```python
from build123d import *

# Parameters (mm, degrees)
F1_DEPTH = 2.54


with BuildPart() as f1:
    # F0 (on Front) → F1 (new body)
    with BuildSketch(Plane.XZ):
        with BuildLine():
            ThreePointArc((7.738306, -7.057663), (9.765713, -3.784552), (10.473394, 0))
            ThreePointArc((10.473394, 0), (9.627005, 4.124653), (7.224635, 7.582653))
            ThreePointArc((7.224635, 7.582653), (0, 10.473394), (-7.224635, 7.582653))
            ThreePointArc((-7.224635, 7.582653), (-10.466954, 0.367244), (-7.738306, -7.057663))
            ThreePointArc((-7.738306, -7.057663), (0, -10.473394), (7.738306, -7.057663))
        make_face()
        with BuildLine():
            Line((-2.152094, -7.214504), (0, -2.595979))
            Line((0, -2.595979), (2.144959, -7.214504))
            ThreePointArc((2.144959, -7.214504), (-0.003567, -7.636494), (-2.152094, -7.214504))
        make_face(mode=Mode.SUBTRACT)
        with BuildLine():
            ThreePointArc((-3.384339, -6.653862), (-6.683961, -3.233143), (-7.223777, 1.488871))
            Line((-7.223777, 1.488871), (-3.384339, -6.653862))
        make_face(mode=Mode.SUBTRACT)
        with BuildLine():
            Line((3.492318, -6.653862), (7.286586, 1.488871))
            ThreePointArc((7.286586, 1.488871), (6.822869, -3.250425), (3.492318, -6.653862))
        make_face(mode=Mode.SUBTRACT)
        with BuildLine():
            ThreePointArc((-5.957007, 4.418221), (-5.252536, 5.505791), (-4.134786, 6.161323))
            Line((-4.134786, 6.161323), (-1.229617, 0))
            Line((-1.229617, 0), (1.402125, 0))
            Line((1.402125, 0), (4.273116, 6.161323))
            ThreePointArc((4.273116, 6.161323), (5.263901, 5.39392), (6.050396, 4.418221))
            Line((6.050396, 4.418221), (2.601226, -2.98391))
            Line((2.601226, -2.98391), (1.402125, -0.328891))
            Line((1.402125, -0.328891), (-1.229617, -0.328891))
            Line((-1.229617, -0.328891), (-2.466776, -2.98391))
            Line((-2.466776, -2.98391), (-5.957007, 4.418221))
        make_face(mode=Mode.SUBTRACT)
        with BuildLine():
            Line((0, 2.846012), (-1.913186, 7.11832))
            ThreePointArc((-1.913186, 7.11832), (0.103343, 7.357841), (2.119873, 7.11832))
            Line((2.119873, 7.11832), (0, 2.846012))
        make_face(mode=Mode.SUBTRACT)
        with BuildLine():
            ThreePointArc((7.224635, 7.582653), (9.627005, 4.124653), (10.473394, 0))
            ThreePointArc((10.473394, 0), (9.765713, -3.784552), (7.738306, -7.057663))
            Line((7.738306, -7.057663), (17.044773, -4.823679))
            Line((17.044773, -4.823679), (17.261992, -4.200394))
            Line((17.261992, -4.200394), (21.515753, 8.005273))
            Line((21.515753, 8.005273), (9.83273, 7.65978))
            Line((9.83273, 7.65978), (7.224635, 7.582653))
        make_face()
        with BuildLine():
            ThreePointArc((-7.738306, -7.057663), (-10.466954, 0.367244), (-7.224635, 7.582653))
            Line((-7.224635, 7.582653), (-9.815511, 7.65978))
            Line((-9.815511, 7.65978), (-21.421401, 8.005273))
            Line((-21.421401, 8.005273), (-17.155705, -4.200394))
            Line((-17.155705, -4.200394), (-16.937877, -4.823679))
            Line((-16.937877, -4.823679), (-7.738306, -7.057663))
        make_face()
        Polygon((-14.769453, 2.473412), (-14.185613, 4.333009), (-13.477944, 2.473412), (-11.474869, 2.473412), (-13.129719, 1.022873), (-12.338734, -1.062449), (-14.252342, 0.338954), (-15.897308, -1.062449), (-15.132699, 1.022873), (-16.792862, 2.473412), align=None, mode=Mode.SUBTRACT)
        Polygon((11.004867, 10.780503), (9.83273, 7.65978), (21.515753, 8.005273), (17.261992, -4.200394), (44.487608, 2.368847), (50.83166, 10.780503), align=None)
        Polygon((-21.421401, 8.005273), (-9.815511, 7.65978), (-11.012142, 10.780503), (-50.76834, 10.780503), (-44.232576, 2.368847), (-17.155705, -4.200394), align=None)
    extrude(amount=F1_DEPTH)


solid = f1.part
```
The listing builds one solid part. Answer for the finished solid, in the listing's coordinates (mm). A direction names the side the tool comes from. Give positions to 0.01 mm unless a question says otherwise; leave off trailing zeros. Order: outer loops, then holes, each group sorted by start corner. A loop starts at its lowest first (then second) coordinate and runs counter-clockwise, first axis right, second up.
Item 1: Find the intervals of material crossed by probe 1 along X at (y, z) = (-1, 5.75); probe 2 along Z at (x, y) = (6, -0.6); probe 3 along Z at (x, y) = (1.5, -0.6), in increasing order.
From the geometry:
probe 1: x = -46.86 to -4.96, -3.94 to -1.3, 1.44 to 4.08, 4.86 to 47.04
probe 2: z = -8.58 to -4.6, -1.27 to 4.31, 4.5 to 8.58
probe 3: z = -10.37 to -7.43, -5.83 to -0.55, 0.21 to 5.87, 7.24 to 10.37
Item 2: The part is cut by section C-C, the plane x = 29.5. Give the vertices of the cut face in (y, z), and give its area (3 significant figures).
From the geometry:
outline: (-2.54, -1.25) - (0, -1.25) - (0, 10.78) - (-2.54, 10.78) - close
area: 30.6 mm2
Item 3: Given pin 1 Ø10 at (x, z) = (-5.5, -5) entering from +Y; pin 2 Ø0.6 at (x, y) = (-13, -1) entering from -Z, each flat-ended and moving along its own axis, determine where each tip first touches the part or whether it passes through.
From the geometry:
pin 1: stops at y = 0
pin 2: stops at z = -5.85
Item 4: For a pull along Z with two mould halves and no side action, classify faces 4 (the face through (-15.951, -1.252, 1.738)), 5 (the face through (31, -1, 10.781)), 6 (the face through (-1, -2.54, 3)), 7 (the face through (12.326, -1.252, -5.956)) as pulls with the +Z half, pulls with the -Z half, needs draft (parallel to the pull), parting line crosses it, or undercut.
From the geometry:
face 4: undercut
face 5: pulls with the +Z half
face 6: needs draft
face 7: pulls with the -Z half
Item 5: The part is cut by section D-D, the plane x = -24.5. Give the vertices of the cut face in (y, z), and give its area (3 significant figures).
From the geometry:
outline: (-2.54, -2.42) - (0, -2.42) - (0, 10.78) - (-2.54, 10.78) - close
area: 33.5 mm2
Item 6: The part is cut by section A-A, the plane z = 8.5. Give the vertices of the cut face in (x, y).
From the geometry:
outline: (-49, -2.54) - (-10.14, -2.54) - (-10.14, 0) - (-49, 0) - close; (-6.12, -2.54) - (6.12, -2.54) - (6.12, 0) - (-6.12, 0) - close; (10.15, -2.54) - (49.11, -2.54) - (49.11, 0) - (10.15, 0) - close
Item 7: The part is cut by section B-B, the plane y = -1.2. Count the separate pieces of the cut face and the enclosed holes in it, and give its area (3 significant figures).
From the geometry:
separate pieces: 1
enclosed holes: 6
area: 1,190 mm2
Item 8: Which of the six approach directions +Z, -Z, +X, -X, +Y, -Y give full straight-line access (tool end or side, diameter ignored) to faces 1 (the face through (-31, -1, 10.781)), 2 (the face through (2.8, -1.3, 3)), 3 (the face through (-10.405, -1.252, 9.198))?
From the geometry:
face 1: +Z, +X, -X, +Y, -Y
face 2: +Y, -Y
face 3: +Z, +Y, -Y
